Could you check a few things on this drawing? It's one solid part, dimensions in mm from its lowest x, y, z. A direction names the side the tool comes from. Coordinates: 2 decimals unless noted, no trailing zeros. Order: outer loops, then holes, each group sorted by start corner. A loop starts at its lowest first (then second) coordinate and runs counter-clockwise, first axis right, second up.
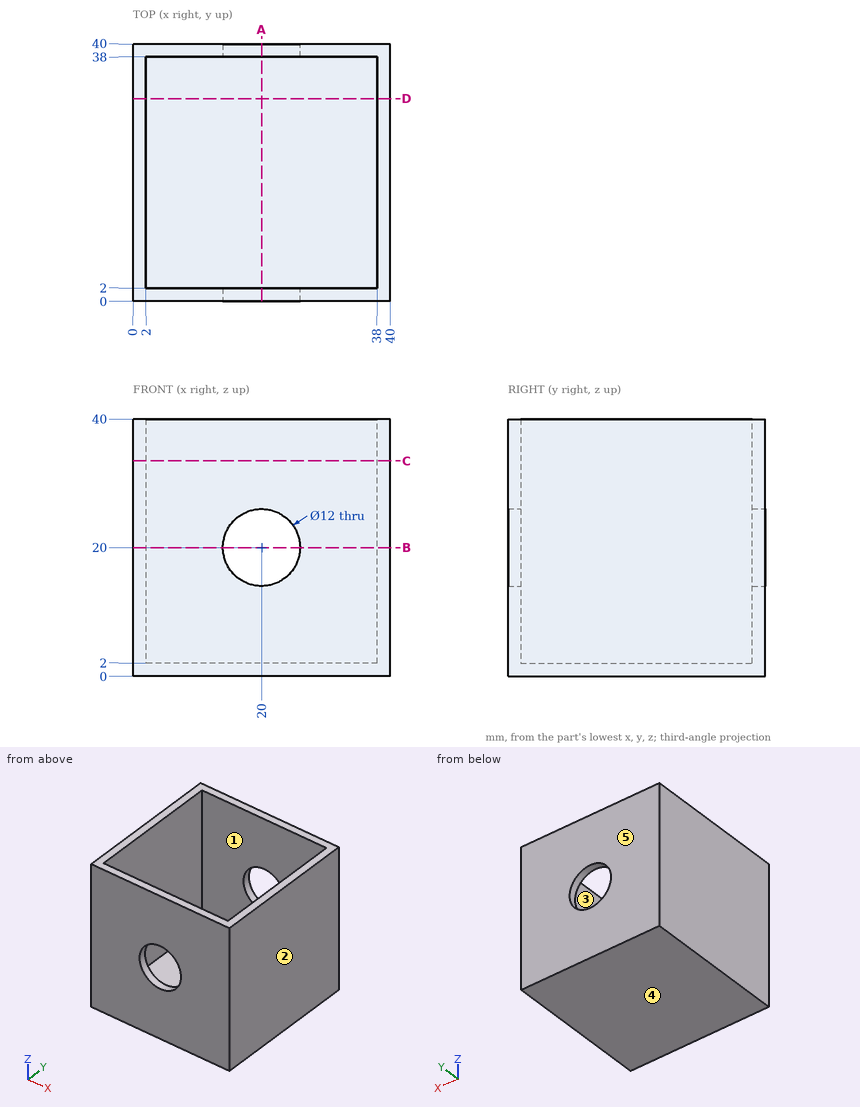
1. Imagine slicing it at C-C on z = 33.5. Please give me the cut outline in (x, y), then the cut area to 3 significant figures.
Completed:
outline: (0, 0) - (40, 0) - (40, 40) - (0, 40) - close; hole (2, 2) - (38, 2) - (38, 38) - (2, 38) - close
area: 304 mm2
2. Imagine slicing it at B-B on z = 20. Please give me the cut outline in (x, y).
Completed:
outline: (0, 0) - (14, 0) - (14, 2) - (2, 2) - (2, 38) - (14, 38) - (14, 40) - (0, 40) - close; (26, 0) - (40, 0) - (40, 40) - (26, 40) - (26, 38) - (38, 38) - (38, 2) - (26, 2) - close
3. Thinking about a two-plate mould opening in Y: for the marked faces 3, 4 and 5, which applies, pulls with the +Y half, pulls with the -Y half, needs draft (parallel to the pull), parting line crosses it, or undercut?
Completed:
face 3: undercut
face 4: needs draft
face 5: pulls with the +Y half
4. On a 3-axis mill with a long thin cutter (end or side, diameter ignored), from which of +Z, -Z, +X, -X, +Y, -Y can I reach the whole of each face in a straight line? I mean the marked faces 1 and 2. Say none if no direction works.
Completed:
face 1: +Z
face 2: +Z, -Z, +X, +Y, -Y
5. Please list where these lines run through material, in increasing order: probe 1 along X at (y, z) = (25, 17.5); probe 2 along Z at (x, y) = (20, 0.6).
Completed:
probe 1: x = 0 to 2, 38 to 40
probe 2: z = 0 to 14, 26 to 40
6. Imagine slicing it at D-D on y = 31.5. Please give me the cut outline in (x, z).
Completed:
outline: (0, 0) - (40, 0) - (40, 40) - (38, 40) - (38, 2) - (2, 2) - (2, 40) - (0, 40) - close
7. Imagine slicing it at A-A on x = 20. Please give me the cut outline in (y, z), then the cut area to 3 significant figures.
Completed:
outline: (0, 0) - (40, 0) - (40, 14) - (38, 14) - (38, 2) - (2, 2) - (2, 14) - (0, 14) - close; (0, 26) - (2, 26) - (2, 40) - (0, 40) - close; (38, 26) - (40, 26) - (40, 40) - (38, 40) - close
area: 184 mm2
8. I'm going to push flat-ended pins straight in: pin 1 (5 mm diameter, centred on x = 34, y = 19.5, fed in from -Z); pin 2 (18 mm diameter, centred on x = 24.5, y = 28.5, fed in from +Z). Where does each tip first touch, or does it pass through?
Completed:
pin 1: stops at z = 0
pin 2: stops at z = 2
